The listing builds one solid part. Answer for the finished solid, in the listing's coordinates (mm). Give positions to 0.01 mm unless a question says otherwise; leave off trailing zeros. Write each loop counter-clockwise with the first axis right and the second up, starting at its lowest first coordinate (ties: lowest second). Pieces come first, ordered by that corner, then holes. Notation, with made-up numbers: (-32.5, 78.25) - (-18.5, 78.25) arc R29 cw to (-18.5, 103.25) - close; hole circle Ø6 at (-34.75, -23). An arc over 180 degrees is marked (long way). One line per question, with ' | ' between items. Start each with the question number.
1. A cutting plane is placed at D-D (y = -66.5). Determine the outline of the cut face in (x, z).
2. Given P1, Ø1, axis at y = -217.5, z = 140, coming from the +X side; P2, Ø8, axis at y = -172.5, z = -84, coming from the -X side; P3, Ø6, axis at y = -156.5, z = -24.5, coming from the +X side, each flat-ended and moving along its own axis, determine where each tip first touches the part or whether it passes through.
3. A cutting plane is placed at B-B (x = 116.5). Determine the outline of the cut face in (y, z).
4. A cutting plane is placed at C-C (z = -40). Determine the outline of the cut face in (x, y).
5. A cutting plane is placed at A-A (y = -141.5). Determine the outline of the cut face in (x, z), then the cut area to 3 significant figures.
6. The mould has two halves that part along Z. Classify faces 1 (the face through (153.67, -174, -2.9)), 2 (the face through (128.21, -129.14, 126.43)), 3 (the face through (86.649, -59.056, 1.098)): +Z half, -Z half, draft (parallel to the pull), parting line (faces both ways), or undercut.
7. Find the intervals of material crossed by L1, parallel to Y at x = 185.5, z = 41.5; L2, parallel to Y at x = 167.5, z = 60.5; L3, parallel to X at y = -196.5, z = -12, in increasing order. Write a range as from..to.
```python
from build123d import *

# Parameters (mm, degrees)
THICKEN1_T1 = 1
THICKEN1_T2 = 1


with BuildPart() as body_1:
    # Sketch2 → Surface-Plane1: a flat surface bounded by the sketch
    with BuildSketch(Plane(origin=(18.304702573, 56.103893903, 84.504712269), x_dir=(-0.3617763934446254, 0.6097357967348626, 0.7052234392916206), z_dir=(-0.8600121206459034, -0.5102736053747404, -1.0969032612691395e-15)), mode=Mode.PRIVATE) as surface_plane1_1_region:
        with BuildLine():
            Line((-158.264155059, -288.964285994), (-88.353199476, -75.303587479))
            ThreePointArc((-88.353199476, -75.303587479), (-154.539912555, -34.528871866), (-194.96195103, 31.873818041))
            Line((-194.96195103, 31.873818041), (-408.99153859, -36.899515812))
            ThreePointArc((-408.99153859, -36.899515812), (-313.925122407, -193.068427437), (-158.264155059, -288.964285994))
        make_face()
    surface_plane1_1 = surface_plane1_1_region.sketch.faces()[0]
    add(Solid.thicken(surface_plane1_1, THICKEN1_T1))
    add(Solid.thicken(surface_plane1_1, -THICKEN1_T2))


solid = body_1.part
```
Determined:
1) outline: (89.89, -88.96) - (92.21, -89.57) - (92.21, 89.57) - (89.89, 88.96) - close
2) P1: x = 182.1 | P2: x = 150.41 | P3: x = 147.39
3) outline: (-111.35, -115.58) - (-107.43, -113.86) - (-107.43, 113.86) - (-111.35, 115.58) - close
4) outline: (83.29, -55.38) - (199.45, -251.15) - (201.17, -250.13) - (85.01, -54.36) - close
5) outline: (134.39, -133.46) - (136.71, -134.07) - (136.71, 134.07) - (134.39, 133.46) - close | area: 622 mm2
6) face 1: draft | face 2: +Z half | face 3: undercut
7) L1: -227.65..-223.73 | L2: -197.31..-193.39 | L3: 167.02..169.35
